The figure shows three views and two pictorial views of one solid part (mm, origin at its lowest corner). Answer the questions. Coordinates: 2 decimals unless noted, no trailing zeros. Loops run counter-clockwise (first coordinate to the right, second up) from the corner with the lowest first, then second, coordinate; pieces in that order, holes last. Notation, with made-up numbers: M 82.5,29 L 124.5,29 A36 cw 124.5,63 Z; hole C 13,73 d5. An arc over 180 degrees is marked long. One line per item, written item: value. Start each with the question number.
1. The part is cut by section A-A (y = 756). Write down the section's boundary in (x, z).
2. Consider probe 1 along Z at (x, y) = (630.5, 952); probe 2 along Z at (x, y) = (82.5, 284). Determine where each line is inside the solid, lowest interval first.
3. Flat-ended cylindrical pins translate along their axes: pin 1 (10 mm diameter, centred on y = 635.5, z = 26.5, fed in from +X); pin 2 (2 mm diameter, centred on x = 502.5, y = 160.5, fed in from +Z). Find the tip coordinate at first contact, or state that the pin passes through.
4. The part is cut by section C-C (z = 65). Write down the section's boundary in (x, y), then the cut area to 3 significant figures.
5. The part is cut by section B-B (x = 516.5). Write down the section's boundary in (y, z), then the cut area to 3 significant figures.
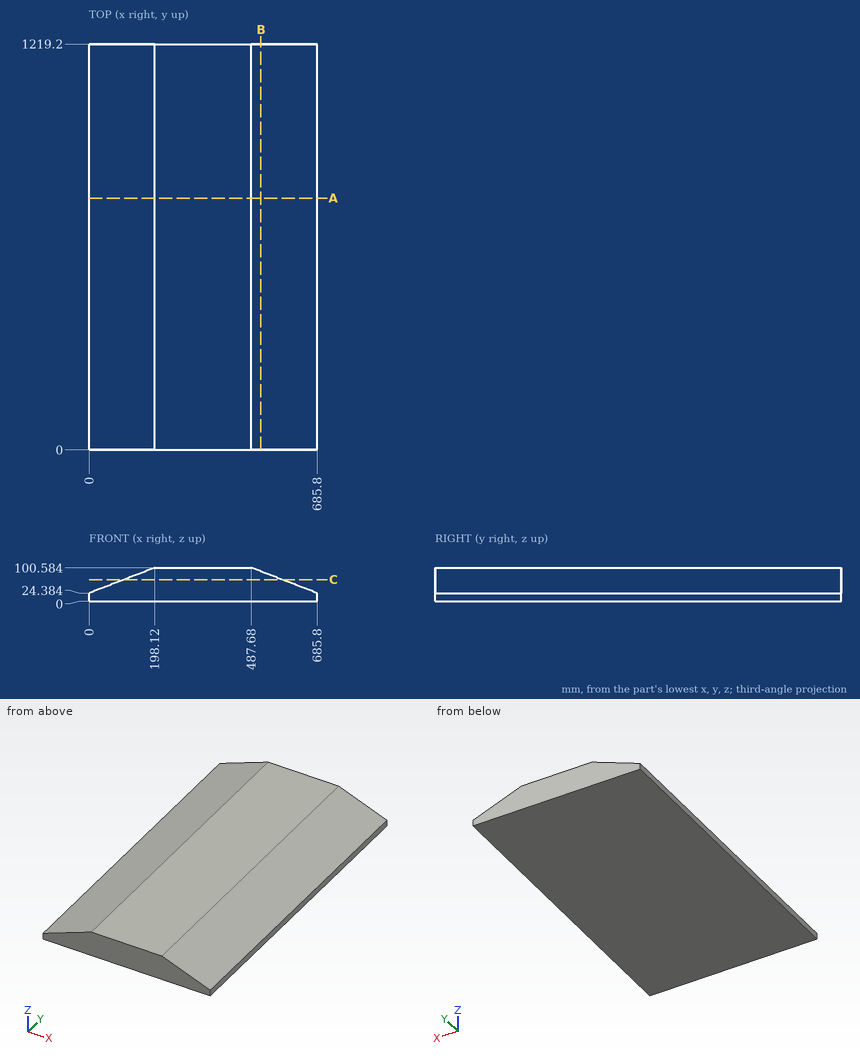
Answer block:
1. outline: M 0,0 L 685.8,0 L 685.8,24.38 L 487.68,100.58 L 198.12,100.58 L 0,24.38 Z
2. probe 1: z = 0 to 45.65
2. probe 2: z = 0 to 56.11
3. pin 1: stops at x = 685.8
3. pin 2: stops at z = 95.27
4. outline: M 105.6,0 L 580.2,0 L 580.2,1219.2 L 105.6,1219.2 Z
4. area: 579,000 mm2
5. outline: M 0,0 L 1219.2,0 L 1219.2,89.5 L 0,89.5 Z
5. area: 109,000 mm2
